Input: part model. Units: mm. Frame: model coordinates. Coordinates: 2 decimals unless noted, no trailing zeros. Loops run counter-clockwise (first coordinate to the right, second up) from the corner with the lowest first, then second, coordinate; pieces in that order, holes last.
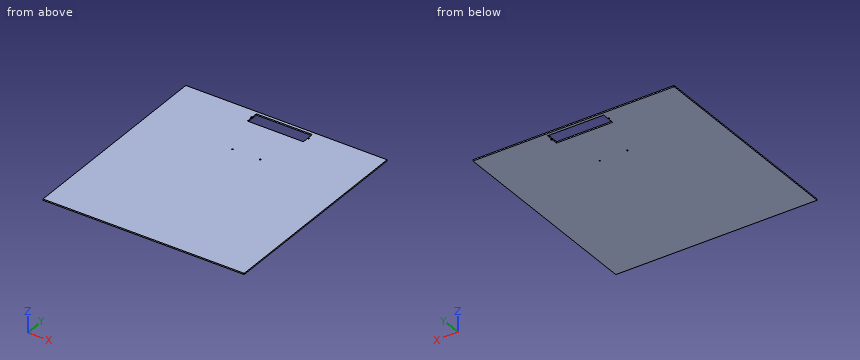
Autodesk Inventor part; units mm, degrees
ref_plane "YZ Plane" through (0, 0, 0) normal (1, 0, 0) x (0, 1, 0)
ref_plane "XZ Plane" through (0, 0, 0) normal (0, 1, 0) x (-1, 0, 0)
ref_plane "XY Plane" through (0, 0, 0) normal (0, 0, 1) x (1, 0, 0)
sketch "Skizze1" plane through (0, 0, 0) normal (0, 0, 1) x (1, 0, 0)
  line L0 (-242, -252) -> (242, -252)
  line L1 (242, -252) -> (242, 252)
  line L2 (242, 252) -> (-242, 252)
  line L3 (-242, 252) -> (-242, -252)
  line L4 (-242, -252) -> (242, 252) construction
  line L5 (242, -252) -> (-242, 252) construction
  line L6 (-67.5, 245) -> (67.5, 245)
  line L7 (67.5, 213) -> (-67.5, 213)
  line L8 (0, 245) -> (0, 213) construction
  line L9 (69.1, 229) -> (-69.1, 229) construction
  line L10 (-69.1, 230.7) -> (-67.5, 230.7)
  line L11 (-69.1, 227.3) -> (-67.5, 227.3)
  line L12 (69.1, 230.7) -> (67.5, 230.7)
  line L13 (69.1, 227.3) -> (67.5, 227.3)
  line L14 (67.5, 245) -> (67.5, 230.7)
  line L15 (67.5, 227.3) -> (67.5, 213)
  arc A0 (69.1, 227.3) -> (69.1, 230.7) centre (69.1, 229) ccw
  arc A1 (-69.1, 230.7) -> (-69.1, 227.3) centre (-69.1, 229) ccw
  line L16 (-67.5, 230.7) -> (-67.5, 245)
  line L17 (-67.5, 213) -> (-67.5, 227.3)
  circle A2 centre (-33.4649, 111.0916) radius 1.7
  circle A3 centre (33.465, 111.0916) radius 1.7
  point P0 (0, 0)
  point P1 (0, 252)
  point P2 (0, 229)
  dimension "d0" = 484
  dimension "d1" = 504
  dimension "d6" = 135
  dimension "d7" = 32
  dimension "d8" = 138.2
  dimension "d10" = 3.4
  dimension "d11" = 117.9083
  dimension "d13" = 3.4
  dimension "d15" = 66.9299
  dimension "d16" = 7
extrude "Extrusion1" add sketch "Skizze1" along normal blind 3
properties part number "Panel Back" material "Polycarbonat, klar"
Item 1: Line query: L1, parallel to Y at x = -15, z = 1.05; L2, parallel to X at y = 112, z = 1.1. Output: solid intervals per line, ascending.
Result:
L1: y = -252 to 213, 245 to 252
L2: x = -242 to -34.9, -32.03 to 32.03, 34.9 to 242
Item 2: Contact query for a flat-ended pin moving along its axis: P1, Ø3, axis at x = -33.46, y = 111.09, coming from the -Z side. Output: stop coordinate, or through.
Result:
P1: passes through
Item 3: Section query A-A (z = 0.65). Output: boundary loops of the cut face in (x, y) (3 decimals), then the cut area to 3 significant figures.
Result:
outline: (-242, -252) - (242, -252) - (242, 252) - (-242, 252) - close; hole (-69.1, 227.3) - (-67.5, 227.3) - (-67.5, 213) - (67.5, 213) - (67.5, 227.3) - (69.1, 227.3) arc R1.7 ccw to (69.1, 230.7) - (67.5, 230.7) - (67.5, 245) - (-67.5, 245) - (-67.5, 230.7) - (-69.1, 230.7) arc R1.7 ccw to start; hole circle Ø3.4 at (-33.465, 111.092); hole circle Ø3.4 at (33.465, 111.092)
area: 240,000 mm2
